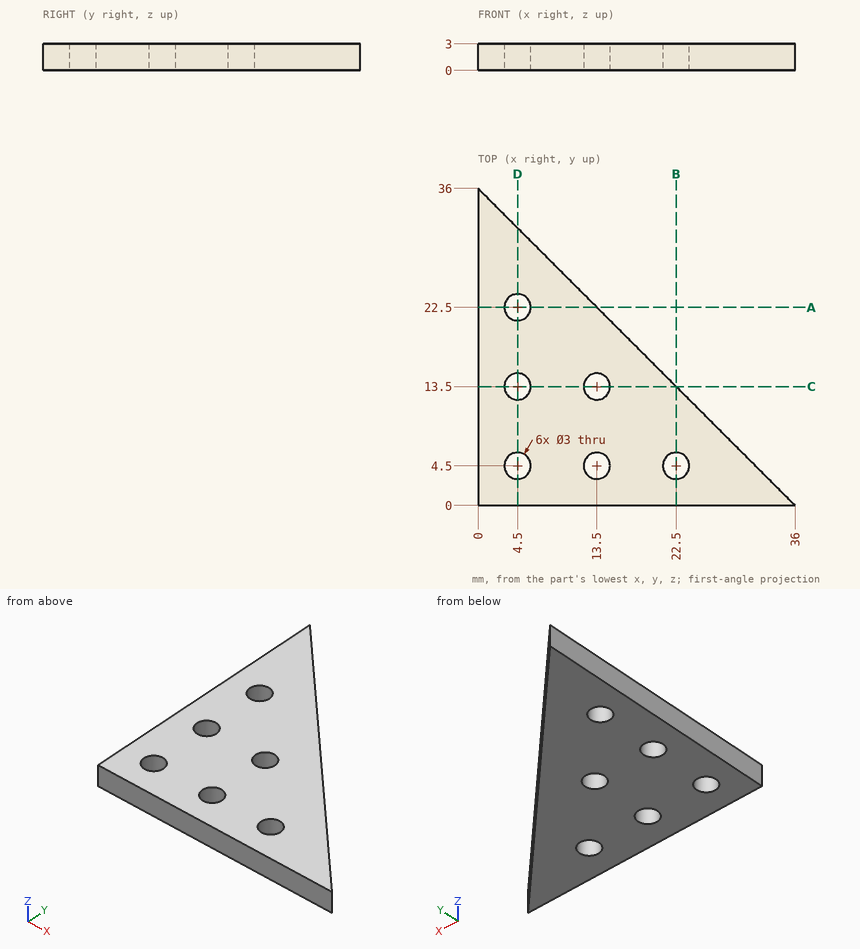
Design review of the part shown in the three views and the two pictorial views. Dimensions are in mm from the part's minimum x, y and z. Give positions to 0.01 mm unless a question says otherwise; leave off trailing zeros. Loops run counter-clockwise (first coordinate to the right, second up) from the corner with the lowest first, then second, coordinate; pieces in that order, holes last. Notation, with made-up numbers: (43.25, -7) -> (49.25, -7) arc R25 cw to (49.25, 23) -> close; hole circle Ø9 at (-5.75, 78.25). An arc over 180 degrees is marked (long way). Write each question's results on one line, items separated by ' | '.
Q1. Wall thickness on L1, parallel to X at y = 13.5, z = 1.4; L2, parallel to Y at x = 4.5, z = 1.9: over which ranges is each line inside the solid? List them lowest first.
Reply:
L1: x = 0 to 3, 6 to 12, 15 to 22.5 | L2: y = 0 to 3, 6 to 12, 15 to 21, 24 to 31.5
Q2. For pin 1 Ø1.5 at (y, z) = (25.5, 2) entering from +X; pin 2 Ø3.5 at (x, y) = (13.5, 4.5) entering from -Z; pin 3 Ø2.5 at (x, y) = (4.5, 22.5) entering from -Z, all flat-tipped, find the tip position at first contact; note any pin that passes through.
Reply:
pin 1: stops at x = 11.25 | pin 2: stops at z = 0 | pin 3: passes through
Q3. Take a section at A-A, the plane y = 22.5. Write out the cut boundary in (x, z).
Reply:
outline: (0, 0) -> (3, 0) -> (3, 3) -> (0, 3) -> close; (6, 0) -> (13.5, 0) -> (13.5, 3) -> (6, 3) -> close
Q4. Take a section at D-D, the plane x = 4.5. Write out the cut boundary in (y, z), plus the area to 3 significant figures.
Reply:
outline: (0, 0) -> (3, 0) -> (3, 3) -> (0, 3) -> close; (6, 0) -> (12, 0) -> (12, 3) -> (6, 3) -> close; (15, 0) -> (21, 0) -> (21, 3) -> (15, 3) -> close; (24, 0) -> (31.5, 0) -> (31.5, 3) -> (24, 3) -> close | area: 67.5 mm²
Q5. Take a section at C-C, the plane y = 13.5. Write out the cut boundary in (x, z).
Reply:
outline: (0, 0) -> (3, 0) -> (3, 3) -> (0, 3) -> close; (6, 0) -> (12, 0) -> (12, 3) -> (6, 3) -> close; (15, 0) -> (22.5, 0) -> (22.5, 3) -> (15, 3) -> close
